```python
from build123d import *

# Parameters (mm, degrees)
MODEL_R             = 1
BOSS_EXTRUDE1_DEPTH = 4
SKETCH2_R           = 2
CUT_EXTRUDE1_DEPTH  = 2


with BuildPart() as part:
    # Model → Boss-Extrude1 (new body)
    with BuildSketch(Plane.XY):
        with BuildLine():
            Line((2, 0), (3, 0))
            Line((3, 0), (3, 5))
            Line((3, 5), (5, 5))
            Line((5, 5), (5, 0))
            Line((5, 0), (11, 0))
            Line((11, 0), (11, 5))
            Line((11, 5), (13, 5))
            Line((13, 5), (13, 0))
            Line((13, 0), (14, 0))
            ThreePointArc((14, 0), (15.414213562, 0.585786438), (16, 2))
            Line((16, 2), (16, 16))
            ThreePointArc((16, 16), (15.414213562, 17.414213562), (14, 18))
            Line((14, 18), (2, 18))
            ThreePointArc((2, 18), (0.585786438, 17.414213562), (0, 16))
            Line((0, 16), (0, 2))
            ThreePointArc((0, 2), (0.585786438, 0.585786438), (2, 0))
        make_face()
        with Locations((4, 15)):
            Circle(MODEL_R, mode=Mode.SUBTRACT)
        with Locations((12, 15)):
            Circle(MODEL_R, mode=Mode.SUBTRACT)
    extrude(amount=BOSS_EXTRUDE1_DEPTH)

    # Sketch2 → Cut-Extrude1 (cut)
    with BuildSketch(Plane.XY.offset(4)):
        with Locations((4, 15)):
            Circle(SKETCH2_R)
        with Locations((12, 15)):
            Circle(SKETCH2_R)
    extrude(amount=-CUT_EXTRUDE1_DEPTH, mode=Mode.SUBTRACT)


solid = part.part
```
Can you work these out from the model? Positions are in its coordinate system, mm. A direction names the side the tool comes from. Coordinates: 2 decimals unless noted, no trailing zeros. Order: outer loops, then holes, each group sorted by start corner. A loop starts at its lowest first (then second) coordinate and runs counter-clockwise, first axis right, second up. Notation, with made-up numbers: (56.5, 55.5) -> (74.5, 55.5) arc R18 cw to (74.5, 68.5) -> close; hole circle Ø7 at (79, 85.25). An arc over 180 degrees is marked (long way). Write each question's results on one line, items separated by ' | '.
Item 1: I'm going to push flat-ended pins straight in: pin 1 Ø1.2 at (x, y) = (11.5, 15.5) entering from +Z; pin 2 Ø1.8 at (x, y) = (12, 15) entering from -Z; pin 3 Ø1 at (x, z) = (12, 1) entering from -Y. Where does each tip first touch, or does it pass through?
Results are:
pin 1: z = 2 | pin 2: through | pin 3: y = 5
Item 2: I want a section at A-A, the plane y = 4.25. Write out the boundary of the cut face in (x, z).
Results are:
outline: (0, 0) -> (3, 0) -> (3, 4) -> (0, 4) -> close; (5, 0) -> (11, 0) -> (11, 4) -> (5, 4) -> close; (13, 0) -> (16, 0) -> (16, 4) -> (13, 4) -> close
Item 3: I want a section at B-B, the plane x = 4. Write out the boundary of the cut face in (y, z).
Results are:
outline: (5, 0) -> (14, 0) -> (14, 2) -> (13, 2) -> (13, 4) -> (5, 4) -> close; (16, 0) -> (18, 0) -> (18, 4) -> (17, 4) -> (17, 2) -> (16, 2) -> close
Item 4: If I drill on line 1 along X through (y, z) = (2.25, 2.15); line 2 along Y through (x, z) = (12, 1.25); line 3 along Y through (x, z) = (5.75, 3.25), over which ranges is the centre line in solid material (lowest first)?
Results are:
line 1: 0 to 3, 5 to 11, 13 to 16 | line 2: 5 to 14, 16 to 18 | line 3: 0 to 14.03, 15.97 to 18
Item 5: If we mould it in two halves opening along X, with no side actions, what happens to faces 4 (the face through (8, 9, 4)), 5 (the face through (4, 17, 3)), 6 (the face through (15.43, 17.4, 1.97))? For each: +X half, -X half, draft (parallel to the pull), parting line (faces both ways), or undercut.
Results are:
face 4: draft | face 5: undercut | face 6: +X half
Item 6: Which directions (+Z, -Z, +X, -X, +Y, -Y) give clear straight access to the entire face, cutting with the end or side of a thin tool? Please do faces 1 (the face through (13, 14, 2)), 2 (the face through (11, 2, 2)), 3 (the face through (16, 9, 2)).
Results are:
face 1: +Z | face 2: +Z, -Z, -Y | face 3: +Z, -Z, +X, +Y, -Y
Item 7: I want a section at D-D, the plane y = 15. Write out the boundary of the cut face in (x, z), then the cut area to 3 significant figures.
Results are:
outline: (0, 0) -> (3, 0) -> (3, 2) -> (2, 2) -> (2, 4) -> (0, 4) -> close; (5, 0) -> (11, 0) -> (11, 2) -> (10, 2) -> (10, 4) -> (6, 4) -> (6, 2) -> (5, 2) -> close; (13, 0) -> (16, 0) -> (16, 4) -> (14, 4) -> (14, 2) -> (13, 2) -> close | area: 40.0 mm²
Item 8: I want a section at C-C, the plane z = 1.6. Write out the boundary of the cut face in (x, y).
Results are:
outline: (0, 2) arc R2 ccw to (2, 0) -> (3, 0) -> (3, 5) -> (5, 5) -> (5, 0) -> (11, 0) -> (11, 5) -> (13, 5) -> (13, 0) -> (14, 0) arc R2 ccw to (16, 2) -> (16, 16) arc R2 ccw to (14, 18) -> (2, 18) arc R2 ccw to (0, 16) -> close; hole circle Ø2 at (4, 15); hole circle Ø2 at (12, 15)
